Part model, mm, in its own coordinate system. Round coordinates to 2 decimals unless told otherwise and drop trailing zeros. Loops run counter-clockwise (first coordinate to the right, second up) from the corner with the lowest first, then second, coordinate; pieces in that order, holes last. Notation, with made-up numbers: (21.25, 2) - (52.25, 2) arc R19 cw to (52.25, 39) - close; hole circle Ø11 at (17, 63.5). An arc over 180 degrees is marked (long way). Write each question's results on one line, items separated by ' | '. Start each with the question number.
(1) Drill centre lines: L1, parallel to Y at x = 48, z = 1.9; L2, parallel to Y at x = 32.5, z = 0.7; L3, parallel to Y at x = -32, z = 0.8. Where is each one in solid material? Low to high.
(2) Cut at B-B, the plane x = 32. List the corners of the cut face in (y, z).
(3) Cut at D-D, the plane y = -60. List the corners of the cut face in (x, z), then the cut area to 3 significant figures.
(4) Flat gauge pins, fed straight in: P1, Ø1.8, axis at x = 48, y = -60, coming from the -Z side; P2, Ø0.9, axis at y = 6.5, z = 1, coming from the +X side; P3, Ø5, axis at x = -32, y = 32, coming from the -Z side; P4, Ø1.5, axis at y = 40.5, z = 1.5, coming from the +X side. Where does each tip first touch, or does it go through?
(5) Cut at C-C, the plane z = 1.5. Give the number of separate pieces and of enclosed holes in the cut face, then the cut area to 3 significant figures.
(6) Cut at A-A, the plane y = 32. List the corners of the cut face in (x, z).
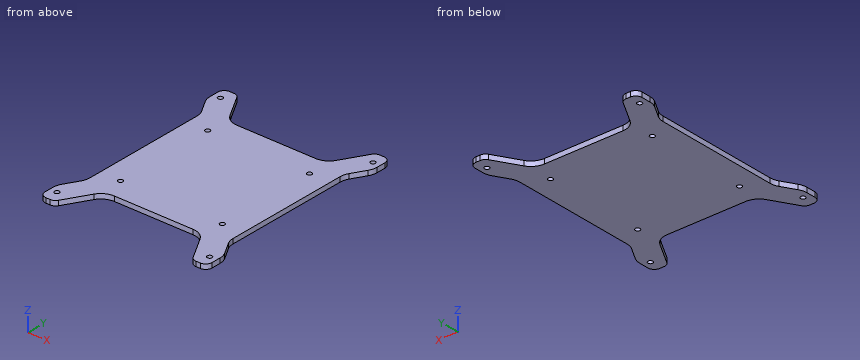
Autodesk Inventor part; units mm, degrees
ref_plane "YZ Plane" through (0, 0, 0) normal (1, 0, 0) x (0, 1, 0)
ref_plane "XZ Plane" through (0, 0, 0) normal (0, 1, 0) x (-1, 0, 0)
ref_plane "XY Plane" through (0, 0, 0) normal (0, 0, 1) x (1, 0, 0)
sketch "Sketch3" plane through (0, 0, 0) normal (0, 0, 1) x (1, 0, 0)
  line L0 (52.5001, -67.5) -> (-52.5001, -67.5)
  line L1 (-52.5001, -67.5) -> (-52.5001, 67.5)
  line L2 (-52.5001, 67.5) -> (52.5001, 67.5)
  line L3 (52.5001, 67.5) -> (52.5001, -67.5)
  circle A0 centre (32, 32) radius 1.5
  circle A1 centre (-32, 32) radius 1.5
  circle A2 centre (-32, -32) radius 1.5
  circle A3 centre (32, -32) radius 1.5
  circle A4 centre (48, 60) radius 1.5
  circle A5 centre (-48, 60) radius 1.5
  circle A6 centre (-48, -60) radius 1.5
  circle A7 centre (48, -60) radius 1.5
  line L4 (30.5, 0) -> (-30.5, 0)
  line L5 (30.5, 45) -> (-30.5, 45)
  line L6 (30.5, 45) -> (43.4898, 67.5)
  line L7 (-30.5, 45) -> (-43.4888, 67.5)
  line L8 (30.5, -45) -> (-30.5, -45)
  line L9 (30.5, -45) -> (43.4898, -67.5)
  line L10 (-30.5, -45) -> (-43.4888, -67.5)
  line L11 (0, 42.0002) -> (0, -42)
  line L12 (45, 42.0002) -> (45, -42)
  line L13 (45, 42.0002) -> (52.5001, 54.9914)
  line L14 (45, -42) -> (52.5001, -54.9922)
  line L15 (-45, 42.0002) -> (-45, -42)
  line L16 (-45, 42.0002) -> (-52.5001, 54.9914)
  line L17 (-45, -42) -> (-52.5001, -54.9922)
extrude "Extrusion2" add sketch "Sketch3" along normal blind 3
fillet "Fillet2" radius 4 4 edges at (-52.5001, 67.5, 1.5) (52.5001, 67.5, 1.5) (52.5001, -67.5, 1.5) (-52.5001, -67.5, 1.5)
extrude "Extrusion3" cut sketch "Sketch3" along normal blind 10 contours L0 L10 L8 L9 | L14 L12 L13 L3 | L1 L16 L15 L17 | L6 L5 L7 L2
fillet "Fillet3" radius 10 8 edges at (30.5, 45, 1.5) (-30.5, 45, 1.5) (30.5, -45, 1.5) (-30.5, -45, 1.5) (-52.5001, 54.9914, 1.5) (52.5001, -54.9922, 1.5) (-52.5001, -54.9922, 1.5) (52.5001, 54.9914, 1.5)
fillet "Fillet4" radius 10 4 edges at (45, 42.0002, 1.5) (45, -42, 1.5) (-45, -42, 1.5) (-45, 42.0002, 1.5)
fillet "Fillet5" radius 4 4 edges at (43.4898, 67.5, 1.5) (-43.4888, 67.5, 1.5) (43.4898, -67.5, 1.5) (-43.4888, -67.5, 1.5)
properties part number "GPS - mount v2"
A:
1) L1: -67.5 to -61.5, -58.5 to -47.2, 47.2 to 58.5, 61.5 to 67.5 | L2: -48.71 to -33.41, -30.59 to 30.59, 33.41 to 48.71 | L3: -48.14 to -33.5, -30.5 to 30.5, 33.5 to 48.14
2) outline: (-48.14, 0) - (-33.5, 0) - (-33.5, 3) - (-48.14, 3) - close; (-30.5, 0) - (30.5, 0) - (30.5, 3) - (-30.5, 3) - close; (33.5, 0) - (48.14, 0) - (48.14, 3) - (33.5, 3) - close
3) outline: (-52.5, 0) - (-49.5, 0) - (-49.5, 3) - (-52.5, 3) - close; (-46.5, 0) - (-39.16, 0) - (-39.16, 3) - (-46.5, 3) - close; (39.16, 0) - (46.5, 0) - (46.5, 3) - (39.16, 3) - close; (49.5, 0) - (52.5, 0) - (52.5, 3) - (49.5, 3) - close | area: 62.0 mm2
4) P1: through | P2: x = 45 | P3: z = 0 | P4: x = 45.19
5) separate pieces: 1 | enclosed holes: 8 | area: 9,340 mm2
6) outline: (-45, 0) - (-33.5, 0) - (-33.5, 3) - (-45, 3) - close; (-30.5, 0) - (30.5, 0) - (30.5, 3) - (-30.5, 3) - close; (33.5, 0) - (45, 0) - (45, 3) - (33.5, 3) - close
